Source: CAD feature listing. Evaluate the final solid. Frame: model axes, mm. Give positions to 0.01 mm unless a question says otherwise; leave off trailing zeros. Order: outer loops, then holes, each group sorted by start corner. A loop starts at its lowest first (then second) coordinate and runs counter-clockwise, first axis right, second up. Notation, with made-up numbers: (-40, 30.5) - (15, 30.5) arc R13 cw to (15, 52.5) - close; hole circle Ø11 at (17.5, 69). An arc over 180 degrees is marked (long way). One line per item, written item: value. Start each with the question number.
from build123d import *

# Parameters (mm, degrees)
ENL_V_MAT_EXTRU_5_DEPTH      = 51.179677161
ENL_V_MAT_EXTRU_5_DEPTH_BACK = 51.179677161
ESQUISSE6_R                  = 1.25
ENL_V_MAT_EXTRU_7_DEPTH      = 51.179677173
ENL_V_MAT_EXTRU_7_DEPTH_BACK = 51.179677173
ESQUISSE8_W                  = 6
ESQUISSE8_H                  = 0.8


with BuildPart() as part:
    # Esquisse1 → Révolution3 (revolve)
    with BuildSketch(Plane.XY, mode=Mode.PRIVATE) as r_volution3_sk:
        Polygon((38.5, 3), (38.5, 1), (47.5, 1), (47.5, 3), (50, 3), (50, 0), (0, 0), (0, 3), (8, 3), (8, 2.5), (9, 2.5), (9, 3), align=None)
    revolve(r_volution3_sk.sketch.rotate(Axis((0, 0, 0), (1, 0, 0)), 90), axis=Axis((0, 0, 0), (1, 0, 0)))

    # Esquisse6 → Enlèv. mat.-Extru.5 (cut, two sides: drawn at the far end of the back side and taken through both)
    with BuildSketch(Plane.XY.offset(-ENL_V_MAT_EXTRU_5_DEPTH_BACK)):
        with Locations((3, 0)):
            Circle(ESQUISSE6_R)
    extrude(amount=ENL_V_MAT_EXTRU_5_DEPTH + ENL_V_MAT_EXTRU_5_DEPTH_BACK, mode=Mode.SUBTRACT)

    # Esquisse8 → Enlèv. mat.-Extru.7 (cut, two sides: drawn at the far end of the back side and taken through both)
    with BuildSketch(Plane(origin=(0, 0, 0), x_dir=(1, 0, 0), z_dir=(0, 1, 0)).offset(-ENL_V_MAT_EXTRU_7_DEPTH_BACK)):
        with Locations((3, 0.4)):
            Rectangle(ESQUISSE8_W, ESQUISSE8_H)
        with Locations((3, -0.4)):
            Rectangle(ESQUISSE8_W, ESQUISSE8_H)
    extrude(amount=ENL_V_MAT_EXTRU_7_DEPTH + ENL_V_MAT_EXTRU_7_DEPTH_BACK, mode=Mode.SUBTRACT)


solid = part.part
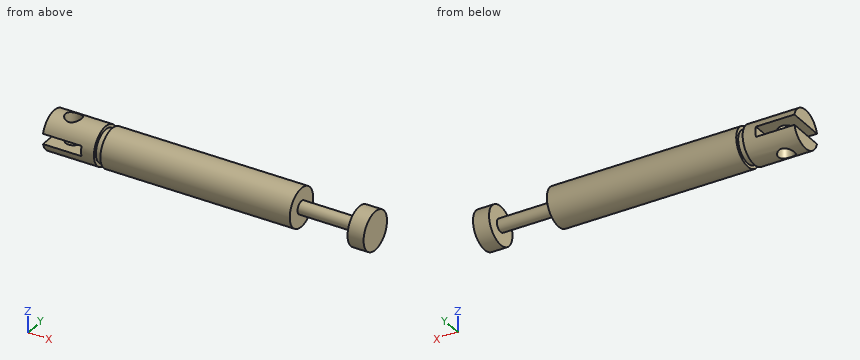
1. Section A-A on y = 0. Count the separate pieces of the cut face and the enclosed holes in it, then the cut area to 3 significant figures.
2. Contact query for flat-ended pins moving along their axis: pin 1 Ø0.5 at (y, z) = (0, 0) entering from -X; pin 2 Ø1 at (x, z) = (30, -1.5) entering from -Y. Output: stop coordinate, or through.
3. Section B-B on z = 0. Return the cut outline in (x, y), then the cut area to 3 significant figures.
4. Section C-C on x = 5. Return the cut outline in (y, z), then the cut area to 3 significant figures.
5. Section D-D on x = 22.5. Return the cut outline in (y, z), then the cut area to 3 significant figures.
6. Ray query, L1, parallel to X at y = 0, z = -2.1; L2, parallel to X at y = 1.5, z = 2.25; L3, parallel to X at y = 1.75, z = 1.25. Return the intervals inside material, ascending.
Data:
1. separate pieces: 3
1. enclosed holes: 0
1. area: 242 mm2
2. pin 1: stops at x = 6
2. pin 2: stops at y = -2.83
3. outline: (6, -3) - (8, -3) - (8, -2.5) - (9, -2.5) - (9, -3) - (38.5, -3) - (38.5, -1) - (47.5, -1) - (47.5, -3) - (50, -3) - (50, 3) - (47.5, 3) - (47.5, 1) - (38.5, 1) - (38.5, 3) - (9, 3) - (9, 2.5) - (8, 2.5) - (8, 3) - (6, 3) - close
3. area: 227 mm2
4. outline: (-2.89, -0.8) arc R3 ccw to (2.89, -0.8) - close; (-2.89, 0.8) - (2.89, 0.8) arc R3 ccw to start
4. area: 18.8 mm2
5. outline: circle Ø6 at (0, 0)
5. area: 28.3 mm2
6. L1: x = 0 to 1.75, 4.25 to 38.5, 47.5 to 50
6. L2: x = 0 to 8, 9 to 38.5, 47.5 to 50
6. L3: x = 0 to 38.5, 47.5 to 50
